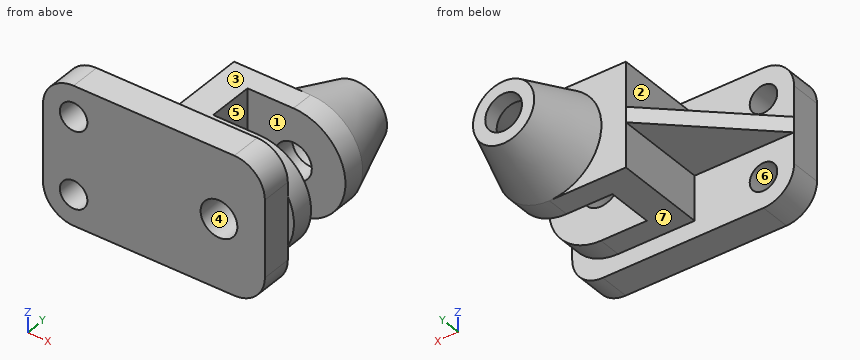
from build123d import *

# Parameters (mm, degrees)
SKETCH1_W           = 145
SKETCH1_H           = 90
SKETCH1_R           = 9
BOSS_EXTRUDE1_DEPTH = 20
FILLET2_R           = 20
BOSS_EXTRUDE3_DEPTH = 60
CUT_EXTRUDE1_START  = -45
CUT_EXTRUDE1_DEPTH  = 30
RIB4_REACH          = 121.487
SKETCH8_WALL_W      = 329.433924144
SKETCH8_WALL_H      = 10
SKETCH18_R          = 12
CUT_EXTRUDE2_DEPTH  = 150.255653159


with BuildPart() as part:
    # Sketch1 → Boss-Extrude1 (new body)
    with BuildSketch(Plane(origin=(0, 0, 0), x_dir=(1, 0, 0), z_dir=(0, 1, 0))):
        Rectangle(SKETCH1_W, SKETCH1_H)
        with Locations(Location((-52.5, 25, 0), (0, 0, 270))):
            Circle(SKETCH1_R, mode=Mode.SUBTRACT)
        with Locations(Location((-52.5, -25, 0), (0, 0, 270))):
            Circle(SKETCH1_R, mode=Mode.SUBTRACT)
    extrude(amount=BOSS_EXTRUDE1_DEPTH)

    # Fillet2
    fillet2_edges = [part.edges().sort_by_distance(p)[0] for p in [
        (72.5, 10, 45),
        (-72.5, 10, 45),
        (-72.5, 10, -45),
        (72.5, 10, -45),
    ]]
    fillet(fillet2_edges, radius=FILLET2_R)

    # Sketch2 → Boss-Extrude3 (add)
    with BuildSketch(Plane(origin=(0, 20, 0), x_dir=(1, 0, 0), z_dir=(0, 1, 0))):
        with BuildLine():
            Line((-7.5, 34), (-7.5, -34))
            Line((-7.5, -34), (42.5, -34))
            ThreePointArc((42.5, -34), (76.5, 0), (42.5, 34))
            Line((42.5, 34), (-7.5, 34))
        make_face()
    extrude(amount=BOSS_EXTRUDE3_DEPTH)

    # Sketch3 → Cut-Extrude1 (cut)
    with BuildSketch(Plane(origin=(0, 80, 0), x_dir=(1, 0, 0), z_dir=(0, 1, 0)).offset(CUT_EXTRUDE1_START)):
        with BuildLine():
            Line((42.5, 34), (12.5, 34))
            Line((12.5, 34), (12.5, -34))
            Line((12.5, -34), (42.5, -34))
            ThreePointArc((42.5, -34), (76.5, 0), (42.5, 34))
        make_face()
    extrude(amount=CUT_EXTRUDE1_DEPTH, mode=Mode.SUBTRACT)

    # Sketch8 wall → Rib4 (add, up to next)
    with BuildSketch(Plane(origin=(-40, 50, 0), x_dir=(-0.734803444627, -0.678280102733, 0), z_dir=(0.678280102733, -0.734803444627, 0)), mode=Mode.PRIVATE) as rib4_sk1:
        Rectangle(SKETCH8_WALL_W, SKETCH8_WALL_H)
    rib4_tool1 = extrude(rib4_sk1.sketch, amount=RIB4_REACH, mode=Mode.PRIVATE) - part.part
    add(rib4_tool1.solids().sort_by_distance((-40, 50, 0))[0])

    # Sketch17 → Revolve-Thin1 (revolve)
    with BuildSketch(Plane(origin=(42.5, 0, 0), x_dir=(0, 0, -1), z_dir=(1, 0, 0))):
        Polygon((0, 80), (0, 120), (20, 120), (34, 80), (24.561416436, 76.696495753), (12.90518995, 110), (10, 110), (10, 80), align=None)
    revolve(axis=Axis((42.5, 80, 0), (0, 1, 0)))

    # Sketch18 → Cut-Extrude2 (cut, through all)
    with BuildSketch(Plane(origin=(0, 120, 0), x_dir=(1, 0, 0), z_dir=(0, 1, 0))):
        with Locations(Location((42.5, 0, 0), (0, 0, 270))):
            Circle(SKETCH18_R)
    extrude(amount=-CUT_EXTRUDE2_DEPTH, mode=Mode.SUBTRACT)


solid = part.part
Work out the finished part from the listing and answer in its coordinate system (mm). Face numbers are marked on the shaded views. A direction names the side the tool comes from. Coordinates: 2 decimals unless noted, no trailing zeros. Order: outer loops, then holes, each group sorted by start corner. A loop starts at its lowest first (then second) coordinate and runs counter-clockwise, first axis right, second up. Notation, with made-up numbers: (31.5, -15.5) - (42.5, -15.5) arc R29 ccw to (42.5, 15.5) - close; hole circle Ø8 at (-31.5, 22.5). An arc over 180 degrees is marked (long way). Put each result on its own line as item: value. Start each with the question number.
1) Find section B-B (y = 12). Give the vertices of the cut face in (x, z), plus the area to 3 significant figures.
2) For the marked faces 1, 2 and 3, determine the directions among +Z, -Z, +X, -X, +Y, -Y from which every point of the face is accessible in a straight line to the end or side of a thin tool.
3) Flat-ended cylindrical pins translate along their axes: pin 1 (5 mm diameter, centred on x = -7, z = 26.5, fed in from -Y); pin 2 (16 mm diameter, centred on x = -52.5, z = 25, fed in from +Y); pin 3 (8 mm diameter, centred on x = -51, y = 34.5, fed in from -Z); pin 4 (12 mm diameter, centred on y = 42.5, z = 16, fed in from -X). Find the tip coordinate at first contact, or state that the pin passes through.
4) For a pull along Z with two mould halves and no side action, classify the marked faces 4, 5, 6 and 7 as released by +Z, released by -Z, zero draft, split by the parting line, or undercut.
5) Find the intervals of material crossed by line 1 (Y direction, x = 32, z = -32.5); line 2 (Z direction, x = -52, y = 14); line 3 (X direction, y = 8, z = -25), in increasing order. Write a range as from..to.
6) Find section A-A (z = 0). State how many separate pieces and enclosed holes the cut face has, plus the area to 3 significant figures.
Results list:
1. outline: (-72.5, -25) arc R20 ccw to (-52.5, -45) - (52.5, -45) arc R20 ccw to (72.5, -25) - (72.5, 25) arc R20 ccw to (52.5, 45) - (-52.5, 45) arc R20 ccw to (-72.5, 25) - close; hole circle Ø18 at (-52.5, -25); hole circle Ø18 at (-52.5, 25); hole circle Ø24 at (42.5, 0)
1. area: 11,700 mm^2
2. face 1: +Z, -Z, +X
2. face 2: +Z, -X, +Y
2. face 3: +Z, +X, -X, +Y
3. pin 1: stops at y = 0
3. pin 2: passes through
3. pin 3: stops at z = -5
3. pin 4: stops at x = -7.5
4. face 4: undercut
4. face 5: zero draft
4. face 6: undercut
4. face 7: released by -Z
5. line 1: y = 0..35, 65..80
5. line 2: z = -45..-33.99, -16.01..16.01, 33.99..45
5. line 3: x = -72.5..-61.5, -43.5..72.5
6. separate pieces: 3
6. enclosed holes: 0
6. area: 7,600 mm^2
